Input: part model. Units: mm. Frame: model coordinates. Round coordinates to 2 decimals unless told otherwise and drop trailing zeros. Return JSON: item names as keys, results as strings. Group by question number.
1) Contact query for a flat-ended pin moving along its axis: P1, Ø12, axis at x = -1, z = -217.5, coming from the -Y side. Output: stop coordinate, or through.
2) Material intervals for line 1 (Y direction, x = -27, z = -116.5); line 2 (Y direction, x = 11.5, z = -155), sorted ascending. Write a range as from..to.
3) Section A-A (y = 5). Count the separate pieces of the cut face and the enclosed holes in it, plus the area to 3 significant figures.
from build123d import *

# Parameters (mm, degrees)
BOSS_EXTRUDE1_DEPTH = 300


with BuildPart() as part:
    # Sketch1 → Boss-Extrude1 (new, symmetric)
    with BuildSketch(Plane.XY):
        Polygon((-30, 7.5), (-30, -7.5), (-27, -2.5), (-24, -7.5), (-21, -2.5), (-18, -7.5), (-15, -2.5), (-12, -7.5), (-9, -2.5), (-6, -7.5), (-3, -2.5), (0, -7.5), (3, -2.5), (6, -7.5), (9, -2.5), (12, -7.5), (15, -2.5), (18, -7.5), (21, -2.5), (24, -7.5), (27, -2.5), (30, -7.5), (30, 7.5), (27, 2.5), (24, 7.5), (21, 2.5), (18, 7.5), (15, 2.5), (12, 7.5), (9, 2.5), (6, 7.5), (3, 2.5), (0, 7.5), (-3, 2.5), (-6, 7.5), (-9, 2.5), (-12, 7.5), (-15, 2.5), (-18, 7.5), (-21, 2.5), (-24, 7.5), (-27, 2.5), align=None)
    extrude(amount=BOSS_EXTRUDE1_DEPTH, both=True)


solid = part.part
Returned:
{
 "1": {"P1": "stops at y = -7.5"},
 "2": {"line 1": "y = -2.5..2.5", "line 2": "y = -6.67..6.67"},
 "3": {"separate pieces": "11", "enclosed holes": "0", "area": "18,000 mm^2"}
}
